from build123d import *

# Parameters (mm, degrees)
SKETCH1_W           = 88.9
SKETCH1_H           = 12.7
SKETCH1_R           = 3.81
BOSS_EXTRUDE1_DEPTH = 7.62
SKETCH2_W           = 58.42
SKETCH2_H           = 12.7
BOSS_EXTRUDE2_DEPTH = 137.16
BOSS_EXTRUDE3_DEPTH = 12.7
SKETCH4_R           = 15.24
CUT_EXTRUDE1_DEPTH  = 12.7
CUT_EXTRUDE2_REACH  = 14.7
SKETCH5_W           = 53.34
SKETCH5_H           = 5.08
FILLET1_R           = 2.54
FILLET2_R           = 2.54


with BuildPart() as part:
    # Sketch1 → Boss-Extrude1 (new body)
    with BuildSketch(Plane(origin=(0, 0, 0), x_dir=(1, 0, 0), z_dir=(0, 1, 0))):
        Rectangle(SKETCH1_W, SKETCH1_H)
        with Locations((-38.1, 0)):
            Circle(SKETCH1_R, mode=Mode.SUBTRACT)
        with Locations((38.1, 0)):
            Circle(SKETCH1_R, mode=Mode.SUBTRACT)
    extrude(amount=BOSS_EXTRUDE1_DEPTH)

    # Sketch2 → Boss-Extrude2 (add)
    with BuildSketch(Plane(origin=(0, 7.62, 0), x_dir=(1, 0, 0), z_dir=(0, 1, 0))):
        Rectangle(SKETCH2_W, SKETCH2_H)
    extrude(amount=BOSS_EXTRUDE2_DEPTH)

    # Sketch3 → Boss-Extrude3 (add)
    with BuildSketch(Plane.XY.offset(6.35)):
        with BuildLine():
            Line((29.21, 144.78), (-29.21, 144.78))
            ThreePointArc((-29.21, 144.78), (0, 173.99), (29.21, 144.78))
        make_face()
    extrude(amount=-BOSS_EXTRUDE3_DEPTH)

    # Sketch4 → Cut-Extrude1 (cut)
    with BuildSketch(Plane(origin=(0, 0, -6.35), x_dir=(-1, 0, 0), z_dir=(0, 0, -1))):
        with Locations((0, 144.78)):
            Circle(SKETCH4_R)
    extrude(amount=-CUT_EXTRUDE1_DEPTH, mode=Mode.SUBTRACT)

    # Sketch5 → Cut-Extrude2 (cut, up to next)
    with BuildSketch(Plane.XY.offset(6.35), mode=Mode.PRIVATE) as cut_extrude2_sk1:
        Polygon((-21.440096834, 121.92), (21.440096834, 121.92), (0, 79.039806331), align=None)
    cut_extrude2_tool1 = extrude(cut_extrude2_sk1.sketch, amount=-CUT_EXTRUDE2_REACH, mode=Mode.PRIVATE) & part.part
    add(cut_extrude2_tool1.solids().sort_by_distance((0, 107.626602, 6.35))[0], mode=Mode.SUBTRACT)
    # Sketch5 → Cut-Extrude2 (cut, up to next)
    with BuildSketch(Plane.XY.offset(6.35), mode=Mode.PRIVATE) as cut_extrude2_sk2:
        Polygon((-21.59, 116.540193669), (-1.419903166, 76.2), (-21.59, 35.859806331), align=None)
    cut_extrude2_tool2 = extrude(cut_extrude2_sk2.sketch, amount=-CUT_EXTRUDE2_REACH, mode=Mode.PRIVATE) & part.part
    add(cut_extrude2_tool2.solids().sort_by_distance((-14.866634, 76.2, 6.35))[0], mode=Mode.SUBTRACT)
    # Sketch5 → Cut-Extrude2 (cut, up to next)
    with BuildSketch(Plane.XY.offset(6.35), mode=Mode.PRIVATE) as cut_extrude2_sk3:
        Polygon((0, 73.360193669), (-21.440096834, 30.48), (21.440096834, 30.48), align=None)
    cut_extrude2_tool3 = extrude(cut_extrude2_sk3.sketch, amount=-CUT_EXTRUDE2_REACH, mode=Mode.PRIVATE) & part.part
    add(cut_extrude2_tool3.solids().sort_by_distance((0, 44.773398, 6.35))[0], mode=Mode.SUBTRACT)
    # Sketch5 → Cut-Extrude2 (cut, up to next)
    with BuildSketch(Plane.XY.offset(6.35), mode=Mode.PRIVATE) as cut_extrude2_sk4:
        Polygon((21.59, 116.540193669), (21.59, 35.859806331), (1.419903166, 76.2), align=None)
    cut_extrude2_tool4 = extrude(cut_extrude2_sk4.sketch, amount=-CUT_EXTRUDE2_REACH, mode=Mode.PRIVATE) & part.part
    add(cut_extrude2_tool4.solids().sort_by_distance((14.866634, 76.2, 6.35))[0], mode=Mode.SUBTRACT)
    # Sketch5 → Cut-Extrude2 (cut, up to next)
    with BuildSketch(Plane.XY.offset(6.35), mode=Mode.PRIVATE) as cut_extrude2_sk5:
        with Locations((0, 2.54)):
            Rectangle(SKETCH5_W, SKETCH5_H)
    cut_extrude2_tool5 = extrude(cut_extrude2_sk5.sketch, amount=-CUT_EXTRUDE2_REACH, mode=Mode.PRIVATE) & part.part
    add(cut_extrude2_tool5.solids().sort_by_distance((0, 2.54, 6.35))[0], mode=Mode.SUBTRACT)

    # Fillet1
    fillet1_edges = [part.edges().sort_by_distance(p)[0] for p in [
        (-29.21, 7.62, 0),
        (29.21, 7.62, 0),
    ]]
    fillet(fillet1_edges, radius=FILLET1_R)

    # Fillet2
    fillet2_edges = [part.edges().sort_by_distance(p)[0] for p in [
        (0, 73.360193669, 0),
        (21.440096834, 30.48, 0),
        (-21.440096834, 30.48, 0),
        (21.59, 35.859806331, 0),
        (1.419903166, 76.2, 0),
        (21.59, 116.540193669, 0),
        (-21.59, 35.859806331, 0),
        (-21.59, 116.540193669, 0),
        (-1.419903166, 76.2, 0),
        (21.440096834, 121.92, 0),
        (0, 79.039806331, 0),
        (-21.440096834, 121.92, 0),
    ]]
    fillet(fillet2_edges, radius=FILLET2_R)


solid = part.part
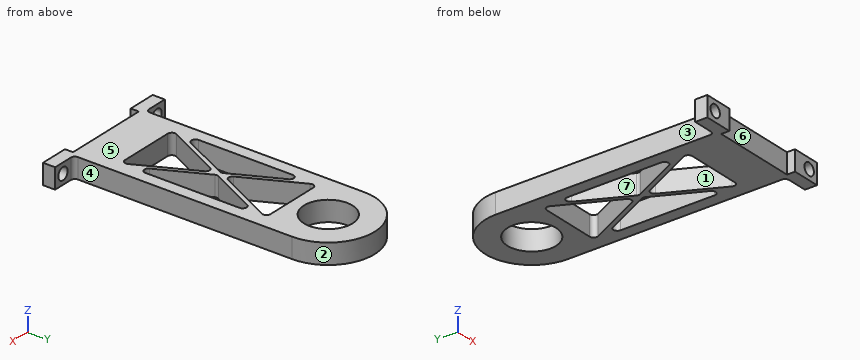
The listing builds one solid part. Answer for the finished solid, in the listing's coordinates (mm). Face numbers are marked on the shaded views. A direction names the side the tool comes from. Give positions to 0.01 mm unless a question says otherwise; leave off trailing zeros. Write each loop counter-clockwise with the first axis right and the second up, starting at its lowest first coordinate (ties: lowest second). Pieces come first, ordered by that corner, then holes.
Item 1: Section C-C, the plane y = 156 is taken. Write down the section's boundary in (x, z).
Item 2: Find the intervals of material crossed by line 1 along X through (y, z) = (5.5, 0); line 2 along X through (y, z) = (68, -4.25); line 3 along Z through (x, y) = (-38.1, 2.5), in increasing order.
Item 3: Which of the six approach directions +Z, -Z, +X, -X, +Y, -Y give full straight-line access (tool end or side, diameter ignored) to the marked faces 1, 2, 3 and 4?
Item 4: Section A-A, the plane x = 38.1 is taken. Write down the section's boundary in (y, z).
Item 5: Determine the mould class of the marked faces 5, 6 and 7 for opening direction Y: released by +Y, released by -Y, zero draft, split by the parting line, or undercut.
Item 6: Flat-ended cylindrical pins translate along their axes: P1, Ø4, axis at y = 82.5, z = -2, coming from the -X side; P2, Ø5, axis at x = 31, y = 77.5, coming from the +Z side; P3, Ø4, axis at x = 4.5, z = -2.5, coming from the -Y side; P4, Ø5, axis at y = 23, z = -2.5, coming from the +X side. Find the tip coordinate at first contact, or state that the pin passes through.
Item 7: Section D-D, the plane z = 0 is taken. Count the separate pieces of the cut face and the enclosed holes in it, plus the area to 3 significant figures.
Item 8: Section B-B, the plane x = 0 is taken. Write down the section's boundary in (y, z), plus the area to 3 significant figures.
Completed:
1. outline: (-26.97, -6.35) - (-10.31, -6.35) - (-10.31, 6.35) - (-26.97, 6.35) - close; (10.31, -6.35) - (26.97, -6.35) - (26.97, 6.35) - (10.31, 6.35) - close
2. line 1: x = -44.45 to -41.91, -34.29 to 34.29, 41.91 to 44.45
2. line 2: x = -29.21 to -21.59, -5.52 to -2.68, 2.68 to 5.52, 21.59 to 29.21
2. line 3: z = -6.35 to -3.81, 3.81 to 6.35
3. face 1: +Z, -Z
3. face 2: +Z, -Z, +Y
3. face 3: +Z, -Z, -X, +Y
3. face 4: +Z, -Z, +X, +Y
4. outline: (0, -6.35) - (7.62, -6.35) - (7.62, -3.81) - (0, -3.81) - close; (0, 3.81) - (7.62, 3.81) - (7.62, 6.35) - (0, 6.35) - close
5. face 5: zero draft
5. face 6: released by -Y
5. face 7: undercut
6. P1: stops at x = -29.21
6. P2: stops at z = 6.35
6. P3: stops at y = 5.08
6. P4: stops at x = 29.21
7. separate pieces: 3
7. enclosed holes: 5
7. area: 5,550 mm2
8. outline: (5.08, -6.35) - (30.48, -6.35) - (30.48, 6.35) - (5.08, 6.35) - close; (70.22, -6.35) - (82.18, -6.35) - (82.18, 6.35) - (70.22, 6.35) - close; (121.92, -6.35) - (129.54, -6.35) - (129.54, 6.35) - (121.92, 6.35) - close; (160.02, -6.35) - (173.99, -6.35) - (173.99, 6.35) - (160.02, 6.35) - close
8. area: 749 mm2
